from build123d import *

# Parameters (mm, degrees)
F1_DEPTH = 63.5
F0_W     = 25.4
F0_H     = 17.7799989994
F2_DEPTH = 25.4
F3_DEPTH = 7.9375
F5_R     = 6.35


with BuildPart() as f1:
    # F0 (on Front) → F1 (new body, symmetric)
    with BuildSketch(Plane.XZ):
        Polygon((-41.275, 9.525), (-41.275, -9.525), (41.275, -9.525), (41.275, -7.9502), (41.275, 9.525), (23.4950010006, 9.525), align=None)
    extrude(amount=F1_DEPTH, both=True)

    # F0 (on Front) → F2 (join, symmetric)
    with BuildSketch(Plane.XZ):
        with BuildLine():
            Line((23.4950010006, 27.0002), (23.4950010006, 9.525))
            Line((23.4950010006, 9.525), (41.275, 9.525))
            Line((41.275, 9.525), (41.275, 27.0002))
            ThreePointArc((41.275, 27.0002), (45.9246798487, 38.2255201513), (57.15, 42.8752))
            Line((57.15, 42.8752), (60.325, 42.8752))
            Line((60.325, 42.8752), (60.325, 60.6551989994))
            Line((60.325, 60.6551989994), (57.15, 60.6551989994))
            ThreePointArc((57.15, 60.6551989994), (33.3523219867, 50.7978780133), (23.4950010006, 27.0002))
        make_face()
        with Locations((73.025, 51.7651994997)):
            Rectangle(F0_W, F0_H)
    extrude(amount=F2_DEPTH, both=True)

    # F0 (on Front) → F3 (join, symmetric)
    with BuildSketch(Plane.XZ):
        with BuildLine():
            add(Edge.make_bspline(
                [(-41.275, 9.525), (-41.1387570202, 33.0824591219), (11.9141172618, 61.0640980303), (57.15, 60.6551989994)],
                knots=[0, 0, 0, 0, 110.9133800527, 110.9133800527, 110.9133800527, 110.9133800527], degree=3))
            Line((-41.275, 9.525), (23.4950010006, 9.525))
            Line((23.4950010006, 9.525), (23.4950010006, 27.0002))
            ThreePointArc((23.4950010006, 27.0002), (33.3523219867, 50.7978780133), (57.15, 60.6551989994))
        make_face()
    extrude(amount=F3_DEPTH, both=True)

    # F0 (on Front) → F4 (revolve)
    with BuildSketch(Plane.XZ):
        Polygon((85.725, 66.675), (85.725, 60.6551989994), (85.725, 42.8752), (85.725, 34.925), (111.125, 34.925), (111.125, 66.675), align=None)
    revolve(axis=Axis((85.725, 0, 50.8), (0, 0, 1)))

    # F5
    f5_edges = [f1.edges().sort_by_distance(p)[0] for p in [
        (41.275, -63.5, 0),
        (-41.275, -63.5, 0),
        (41.275, 63.5, 0),
        (-41.275, 63.5, 0),
    ]]
    fillet(f5_edges, radius=F5_R)


solid = f1.part
The model under review builds one solid part; all positions refer to its coordinate system, in mm. A direction names the side the tool comes from. Coordinates: 2 decimals unless noted, no trailing zeros. Write each loop counter-clockwise with the first axis right and the second up, starting at its lowest first coordinate (ties: lowest second). Pieces come first, ordered by that corner, then holes. Notation, with made-up numbers: (15, 61.25) - (60, 61.25) arc R19 cw to (60, 88.25) - close; hole circle Ø7 at (2, -24). An arc over 180 degrees is marked (long way). Answer as CSV lines item,"result".
(1) We need section B-B (y = 21). Give the boundary of the cut face in (x, z) (3 decimals).
Data:
outline,"(-41.275, -9.525) - (41.275, -9.525) - (41.275, 27) arc R15.875 cw to (57.15, 42.875) - (71.437, 42.875) - (71.437, 34.925) - (100.013, 34.925) - (100.013, 66.675) - (71.437, 66.675) - (71.437, 60.655) - (57.15, 60.655) arc R33.655 ccw to (23.495, 27) - (23.495, 9.525) - (-41.275, 9.525) - close"
(2) For line 1 along Z through (x, y) = (29, -47.5) (3 decimals); line 2 along X through (y, z) = (11.5, 10.5) (3 decimals); line 3 along Y through (x, z) = (-10, 36), list the stretches that pass through material, from the lowest coordinate up. Write a range as [from, to].
Data:
line 1,"z = [-9.525, 9.525]"
line 2,"x = [23.495, 41.275]"
line 3,"y = [-7.94, 7.94]"
(3) Clearance check with flat-ended pins moving along their axes: pin 1 Ø15.5 at (x, z) = (50, 31.5) entering from +Y; pin 2 Ø14.5 at (x, y) = (65.5, -9) entering from -Z (3 decimals); pin 3 Ø3 at (x, z) = (-4.5, 26.5) entering from -Y. State where each tip first meets the part, or that it passes through.
Data:
pin 1,"stops at y = 25.4"
pin 2,"stops at z = 34.925"
pin 3,"stops at y = -7.94"
(4) Tool access review of faces 1 (the cylindrical face through (33.62, 16.55, 51.06)), 2 (the flat face through (47, -25.4, 41)), 3 (the flat face through (60, 2, 42.875)), 4 (the flat face through (23.495, -17, 18)): name each direction out of +Z, -Z, +X, -X, +Y, -Y from which nothing blocks a thin tool from reaching the whole face with its end or side.
Data:
face 1,"+Z, -X, +Y"
face 2,"+Z, +X, -X, -Y"
face 3,"-Z"
face 4,"+Z, -X, -Y"
(5) Mouldability with a two-part tool opening along X and no side actions: class faces 5 (the cylindrical face through (-39.365, -61.689, -0.133)), 6 (the cylindrical face through (45.8, -0.4, 38.1)), 7 (the flat face through (47, 25.4, 41)) as pulls with the +X half, pulls with the -X half, needs draft (parallel to the pull), parting line crosses it, or undercut.
Data:
face 5,"pulls with the -X half"
face 6,"undercut"
face 7,"needs draft"
(6) We need section A-A (y = 49.5). Give the boundary of the cut face in (x, z) (3 decimals), plus the area to 3 significant figures.
Data:
outline,"(-41.275, -9.525) - (41.275, -9.525) - (41.275, 9.525) - (-41.275, 9.525) - close"
area,"1,570 mm2"
(7) We need section C-C (x = 98.5). Give the boundary of the cut face in (y, z) (3 decimals), plus the area to 3 significant figures.
Data:
outline,"(-21.954, 34.925) - (21.954, 34.925) - (21.954, 66.675) - (-21.954, 66.675) - close"
area,"1,390 mm2"
